The model under review builds one solid part; all positions refer to its coordinate system, in mm. A direction names the side the tool comes from. Give positions to 0.01 mm unless a question says otherwise; leave off trailing zeros. Loops run counter-clockwise (first coordinate to the right, second up) from the corner with the lowest first, then second, coordinate; pieces in that order, holes last. Notation, with made-up numbers: M 30,-1 L 71,-1 A17 cw 71,32 Z; hole C -5,2 d7. An arc over 180 degrees is marked long. Put each result on its own line as item: value. Start each with the question number.
from build123d import *

# Parameters (mm, degrees)
SKETCH2_R           = 2.5
BOSS_EXTRUDE1_DEPTH = 25
SKETCH3_R           = 1
CUT_EXTRUDE1_DEPTH  = 25


with BuildPart() as part:
    # Sketch2 → Boss-Extrude1 (new body)
    with BuildSketch(Plane(origin=(0, 0, 0), x_dir=(1, 0, 0), z_dir=(0, 1, 0))):
        with BuildLine():
            Line((0, 33.847554993), (0, -135.452445007))
            ThreePointArc((0, -135.452445007), (7.041241452, -140.016799653), (8.333333333, -131.725665044))
            ThreePointArc((8.333333333, -131.725665044), (5.871290708, -128.354588024), (5, -124.272105119))
            Line((5, -124.272105119), (5, -26.632784894))
            ThreePointArc((5, -26.632784894), (5.871290708, -22.55030199), (8.333333333, -19.179224969))
            ThreePointArc((8.333333333, -19.179224969), (10, -15.452445007), (8.333333333, -11.725665044))
            ThreePointArc((8.333333333, -11.725665044), (5.871290708, -8.354588024), (5, -4.272105119))
            Line((5, -4.272105119), (5, 33.847554993))
            Line((5, 33.847554993), (0, 33.847554993))
        make_face()
        with Locations(Location((5, -15.452445007, 0), (0, 0, 270))):
            Circle(SKETCH2_R, mode=Mode.SUBTRACT)
        with Locations(Location((5, -135.452445007, 0), (0, 0, 270))):
            Circle(SKETCH2_R, mode=Mode.SUBTRACT)
    extrude(amount=BOSS_EXTRUDE1_DEPTH)

    # Sketch3 → Cut-Extrude1 (cut)
    with BuildSketch(Plane(origin=(0, 0, -33.847554993), x_dir=(-1, 0, 0), z_dir=(0, 0, -1))):
        with Locations((-2.5, 10)):
            Circle(SKETCH3_R)
        with Locations((-2.5, 20)):
            Circle(SKETCH3_R)
    extrude(amount=-CUT_EXTRUDE1_DEPTH, mode=Mode.SUBTRACT)


solid = part.part
(1) Draft analysis for pull direction Z (two halves, no side actions). For faces 4 (the cylindrical face through (5.895, 12.325, 128.408)), 5 (the flat face through (0, 12, 50)), 6 (the flat face through (3, 12, -33.848)), state which applies: +Z half, -Z half, draft (parallel to the pull), parting line (faces both ways), or undercut.
(2) To check wall thickness, follow L1, parallel to Y at x = 2.5, z = -22.25; L2, parallel to Z at x = 3.25, y = 23.75; L3, parallel to X at y = 6, z = 55. State the ranges of each line that lie inside material, in increasing order. Write a range as [from, to].
(3) For faces 1 (the cylindrical face through (5.85, 12.32, 22.6)), 2 (the flat face through (5, 12, -15)), 3 (the flat face through (3, 25, 52)), list the 3-axis set-ups (+Z, -Z, +X, -X, +Y, -Y) from which the entire face can be reached by the end or side of a thin tool; tool diameter is ignored.
(4) We need section A-A, the plane y = 14. Write out the cut boundary in (x, z).
(5) Insertion check: pin 1 (6 mm diameter, centred on y = 3, z = 66.5, fed in from +X); pin 2 (4 mm diameter, centred on x = 8.5, y = 16.5, fed in from +Z); pin 3 (4 mm diameter, centred on y = 12.5, z = 9, fed in from +X). Each pin has a flat end and moves straight along its axis. Give the tip position at first contact, or say it passes through.
(6) We need section B-B, the plane z = 109.5. Write out the cut boundary in (x, y), plus the area to 3 significant figures.
Check sheet entries:
1. face 4: undercut
1. face 5: draft
1. face 6: -Z half
2. L1: y = [0, 9], [11, 19], [21, 25]
2. L2: z = [-33.85, 13.67], [17.24, 133.67], [137.24, 140.14]
2. L3: x = [0, 5]
3. face 1: +X, +Y, -Y
3. face 2: -Z, +X, +Y, -Y
3. face 3: +Z, -Z, +X, -X, +Y
4. outline: M 0,-33.85 L 5,-33.85 L 5,4.27 A10 cw 8.33,11.73 A5 ccw 8.33,19.18 A10 cw 5,26.63 L 5,124.27 A10 cw 8.33,131.73 A5 ccw long 0,135.45 Z; hole C 5,15.45 d5; hole C 5,135.45 d5
5. pin 1: stops at x = 5
5. pin 2: stops at z = 140.22
5. pin 3: stops at x = 7.6
6. outline: M 0,0 L 5,0 L 5,25 L 0,25 Z
6. area: 125 mm²
